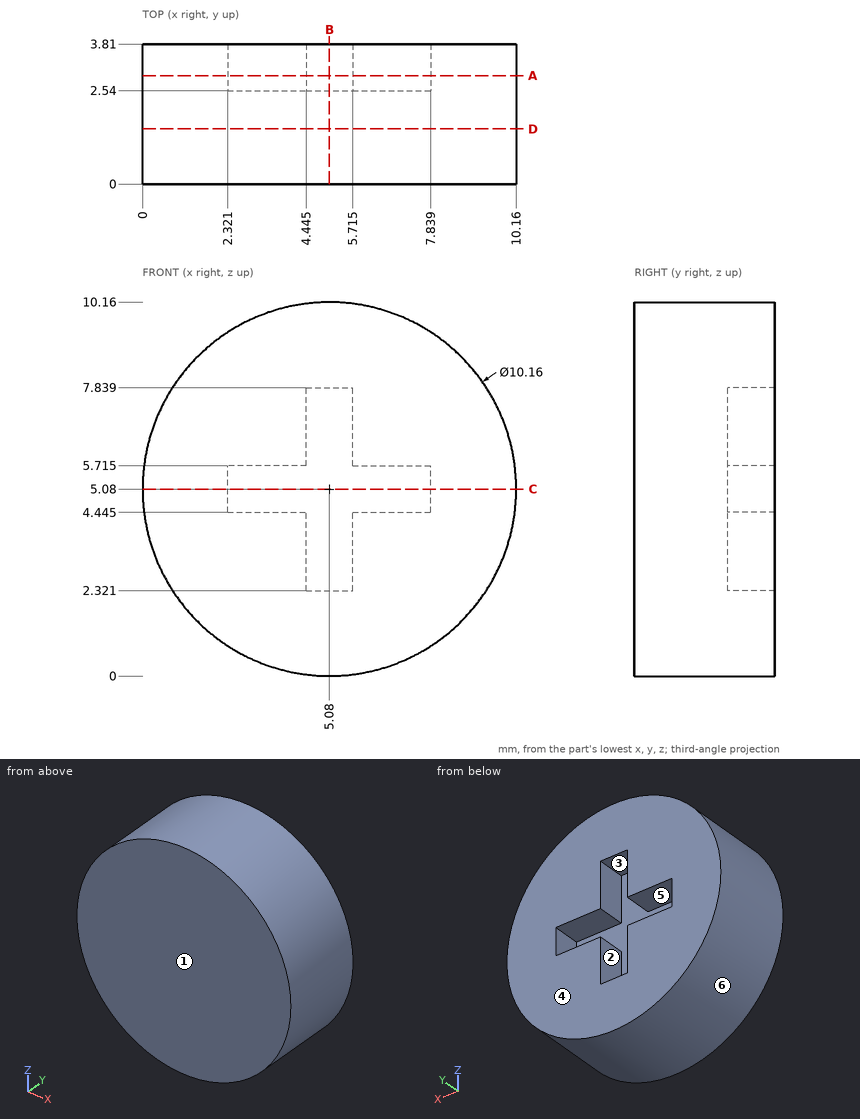
Print and shaded views of the part. All mm, measured from the part's lowest x, y and z. A direction names the side the tool comes from. Give positions to 0.01 mm unless a question says otherwise; leave off trailing zeros. Loops run counter-clockwise (first coordinate to the right, second up) from the corner with the lowest first, then second, coordinate; pieces in that order, holes last. Notation, with made-up numbers: (74, 25) -> (85, 25) arc R10 ccw to (85, 31) -> close; hole circle Ø6 at (10, 84.25). An arc over 180 degrees is marked (long way). One line per question, with ' | ' between items. Start each with the question number.
1) Cut at B-B (x = 5.08). Give the cut face in (y, z).
2) Cut at D-D (y = 1.5). Give the cut face in (x, z).
3) Pin check, flat tips, straight feed: pin 1 (1.4 mm diameter, centred on x = 7, y = 3, fed in from +Z); pin 2 (1.4 mm diameter, centred on x = 3, y = 3, fed in from -Z); pin 3 (0.6 mm diameter, centred on y = 3.5, z = 3.5, fed in from -X); pin 4 (1 mm diameter, centred on x = 4.5, z = 2.5, fed in from -Y). Stop position of each tip, or through.
4) Cut at C-C (z = 5.08). Give the cut face in (x, y), plus the area to 3 significant figures.
5) Cut at A-A (y = 2.95). Give the cut face in (x, z) (3 decimals), plus the area to 3 significant figures.
6) 3-axis set-ups, long thin cutter, end or side, ignore diameter. For the marked faces 1 and 2: which of +Z, -Z, +X, -X, +Y, -Y reach the whole face in a straight line?
7) Two-plate mould, pull along X, no slides. Class the marked faces 3, 4, 5 and 6: released by +X, released by -X, zero draft, split by the parting line, or undercut.
8) Probe L1, parallel to Z at x = 5, y = 3.35; L2, parallel to X at y = 2.15, z = 5; L3, parallel to X at y = 2.6, z = 7.5 (1 decimal). List the from-to ranges inside material, lowest first.
Return value:
1) outline: (0, 0) -> (3.81, 0) -> (3.81, 2.32) -> (2.54, 2.32) -> (2.54, 7.84) -> (3.81, 7.84) -> (3.81, 10.16) -> (0, 10.16) -> close
2) outline: circle Ø10.16 at (5.08, 5.08)
3) pin 1: z = 10.01 | pin 2: z = 0.19 | pin 3: x = 0.16 | pin 4: y = 0
4) outline: (0, 0) -> (10.16, 0) -> (10.16, 3.81) -> (7.84, 3.81) -> (7.84, 2.54) -> (2.32, 2.54) -> (2.32, 3.81) -> (0, 3.81) -> close | area: 31.7 mm^2
5) outline: circle Ø10.16 at (5.08, 5.08); hole (2.321, 4.445) -> (4.445, 4.445) -> (4.445, 2.321) -> (5.715, 2.321) -> (5.715, 4.445) -> (7.839, 4.445) -> (7.839, 5.715) -> (5.715, 5.715) -> (5.715, 7.839) -> (4.445, 7.839) -> (4.445, 5.715) -> (2.321, 5.715) -> close | area: 68.7 mm^2
6) face 1: +Z, -Z, +X, -X, -Y | face 2: +Y
7) face 3: undercut | face 4: zero draft | face 5: undercut | face 6: split by the parting line
8) L1: 0 to 2.32, 7.84 to 10.16 | L2: 0 to 10.16 | L3: 0.6 to 4.4, 5.7 to 9.5
